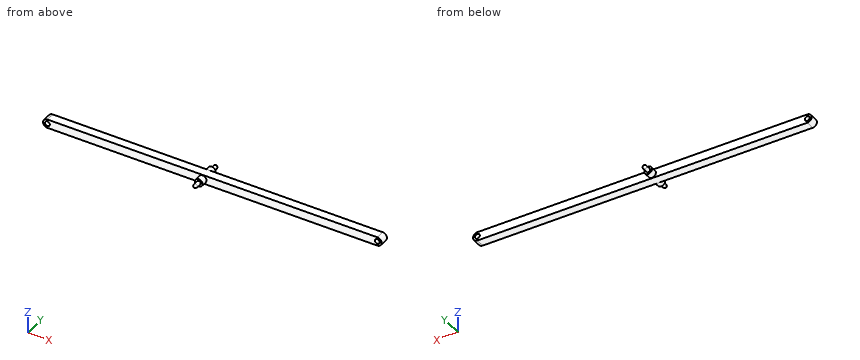
from build123d import *

# Parameters (mm, degrees)
BOSS_EXTRUDE1_DEPTH          = 9
SKETCH2_R                    = 4
BOSS_EXTRUDE2_DEPTH          = 6.5
BOSS_EXTRUDE4_START          = 6.5
SKETCH4_R                    = 4
BOSS_EXTRUDE4_DEPTH          = 6.5
F_5_0_5_DIAMETER_HOLE1_D     = 5
F_5_0_5_DIAMETER_HOLE1_DEPTH = 23


# Read off the part's stored shape, not the designer's step: Boss-Extrude3, Boss-Extrude5
with BuildPart() as part:
    # Sketch1 → Boss-Extrude1 (new body)
    with BuildSketch(Plane(origin=(0, 4.5, 0), x_dir=(1, 0, 0), z_dir=(0, 1, 0))):
        with BuildLine():
            Line((-170, -43.5), (170, -43.5))
            ThreePointArc((170, -43.5), (174.5, -39), (170, -34.5))
            Line((170, -34.5), (-170, -34.5))
            ThreePointArc((-170, -34.5), (-174.5, -39), (-170, -43.5))
        make_face()
    extrude(amount=-BOSS_EXTRUDE1_DEPTH)

    # Sketch2 → Boss-Extrude2 (add)
    with BuildSketch(Plane.XZ.offset(4.5)):
        with Locations(Location((-10, 39, 0), (0, 0, 90))):
            Circle(SKETCH2_R)
    extrude(amount=BOSS_EXTRUDE2_DEPTH)

    # Boss-Extrude3 outline → Boss-Extrude3 (revolve)
    with BuildSketch(Plane(origin=(-10, 0, 39), x_dir=(1, 0, 0), z_dir=(0, 0, 1))):
        with BuildLine():
            ThreePointArc((0, -18.5), (1.414213563, -17.914213562), (2, -16.499999998))
            Line((2, -16.499999998), (2, -11))
            Line((2, -11), (0, -11))
            Line((0, -11), (0, -18.5))
        make_face()
    revolve(axis=Axis((-10, 0, 39), (0, 1, 0)))

    # Sketch4 → Boss-Extrude4 (add)
    with BuildSketch(Plane(origin=(0, 4.5, 0), x_dir=(-1, 0, 0), z_dir=(0, 1, 0)).offset(BOSS_EXTRUDE4_START)):
        with Locations(Location((10, 39, 0), (0, 0, 90))):
            Circle(SKETCH4_R)
    extrude(amount=-BOSS_EXTRUDE4_DEPTH)

    # Boss-Extrude5 outline → Boss-Extrude5 (revolve)
    with BuildSketch(Plane(origin=(-10, 0, 39), x_dir=(1, 0, 0), z_dir=(0, 0, 1))):
        with BuildLine():
            Line((2, 11), (2, 16.499999998))
            ThreePointArc((2, 16.499999998), (1.414213563, 17.914213562), (0, 18.5))
            Line((0, 18.5), (0, 11))
            Line((0, 11), (2, 11))
        make_face()
    revolve(axis=Axis((-10, 0, 39), (0, 1, 0)))

    # Ø5.0 (5) Diameter Hole1
    with Locations(Plane(origin=(0, 4.5, 0), x_dir=(1, 0, 0), z_dir=(0, 1, 0))):
        with Locations((-170, -39), (170, -39)):
            Hole(F_5_0_5_DIAMETER_HOLE1_D / 2, depth=F_5_0_5_DIAMETER_HOLE1_DEPTH)


solid = part.part
Could you check a few things on this model? Use its own coordinates, in mm. Give positions to 0.01 mm unless a question says otherwise; leave off trailing zeros. Order: outer loops, then holes, each group sorted by start corner. A loop starts at its lowest first (then second) coordinate and runs counter-clockwise, first axis right, second up. Notation, with made-up numbers: (72.5, -27.5) - (86.5, -27.5) arc R11 cw to (86.5, -15.5) - close; hole circle Ø9 at (15, -30.5). An arc over 180 degrees is marked (long way). One line per item, written item: value. Start each with the question number.
1. If I drill on probe 1 along X at (y, z) = (2, 39); probe 2 along Z at (x, y) = (170, -0.5); probe 3 along Y at (x, z) = (-52.5, 42.25), over which ranges is the centre line in solid material (lowest first)?
2. Imagine slicing it at C-C on x = 50. List the corners of the cut face in (y, z) for me, plus the area to 3 significant figures.
3. Imagine slicing it at A-A on z = 39. List the corners of the cut face in (x, y) for me.
4. Imagine slicing it at B-B on y = 0. List the corners of the cut face in (x, z) for me, plus the area to 3 significant figures.
5. For P1, Ø4, axis at x = 170, z = 39, coming from the +Y side; P2, Ø2, axis at x = 58.5, z = 37, coming from the +Y side; P3, Ø5, axis at y = 9, z = 38.5, coming from the -X side; P4, Ø1, axis at x = -23.5, z = 37, coming from the -Y side, each with a flat end and sliding along its axis, tell me the tip position at first contact or that it passes through.
Values:
1. probe 1: -174.5 to -172.5, -167.5 to 167.5, 172.5 to 174.5
1. probe 2: 34.5 to 36.5, 41.5 to 43.5
1. probe 3: -4.5 to 4.5
2. outline: (-4.5, 34.5) - (4.5, 34.5) - (4.5, 43.5) - (-4.5, 43.5) - close
2. area: 81.0 mm²
3. outline: (-174.5, -4.5) - (-172.5, -4.5) - (-172.5, 4.5) - (-174.5, 4.5) - close; (-167.5, -4.5) - (-14, -4.5) - (-14, -11) - (-12, -11) - (-12, -16.5) arc R2 ccw to (-8, -16.5) - (-8, -11) - (-6, -11) - (-6, -4.5) - (167.5, -4.5) - (167.5, 4.5) - (-6, 4.5) - (-6, 11) - (-8, 11) - (-8, 16.5) arc R2 ccw to (-12, 16.5) - (-12, 11) - (-14, 11) - (-14, 4.5) - (-167.5, 4.5) - close; (172.5, -4.5) - (174.5, -4.5) - (174.5, 4.5) - (172.5, 4.5) - close
4. outline: (-170, 34.5) - (170, 34.5) arc R4.5 ccw to (170, 43.5) - (-170, 43.5) arc R4.5 ccw to start; hole circle Ø5 at (-170, 39); hole circle Ø5 at (170, 39)
4. area: 3,080 mm²
5. P1: through
5. P2: y = 4.5
5. P3: x = -14
5. P4: y = -4.5
